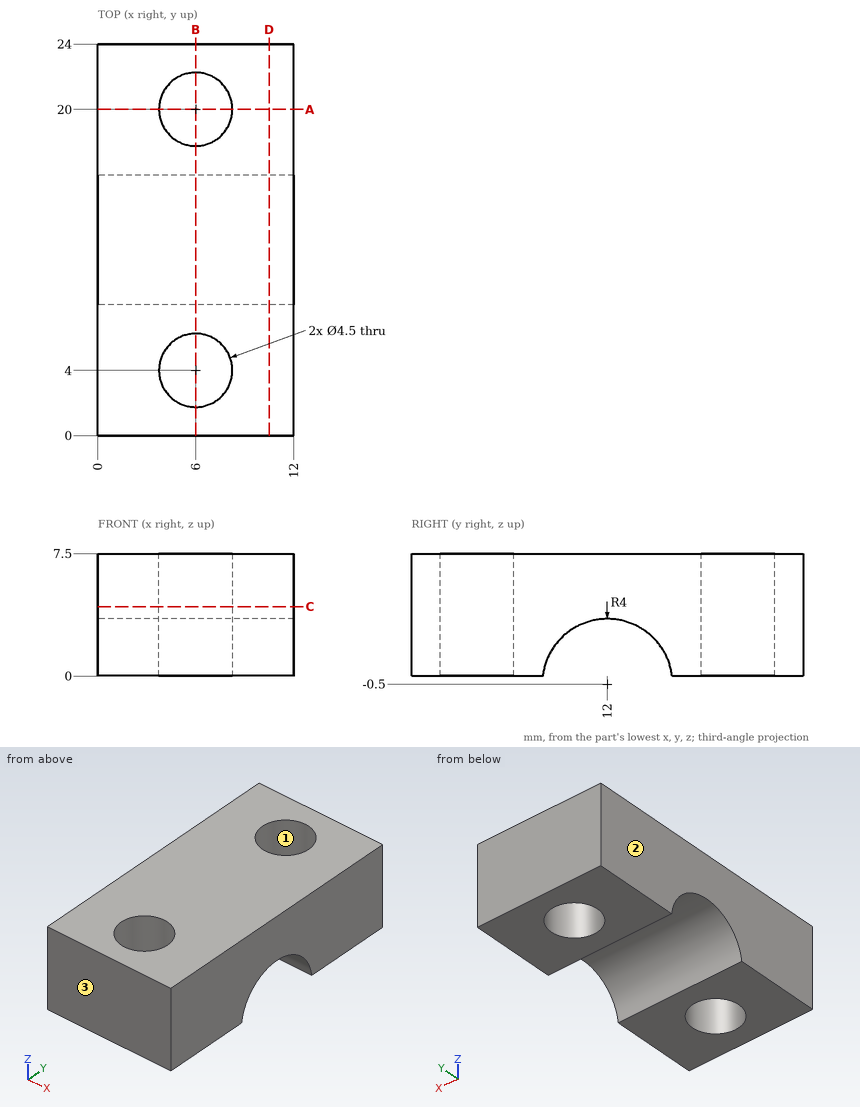
Check sheet for the drawn part. Datum: minimum x, y, z corner. Units: mm. Coordinates: 2 decimals unless noted, no trailing zeros. Order: outer loops, then holes, each group sorted by start corner. A loop starts at its lowest first (then second) coordinate and runs counter-clockwise, first axis right, second up. Notation, with made-up numbers: M -27,49 L -16,49 A12 ccw -16,66 Z; hole C 69,-34.75 d9. An arc over 180 degrees is marked long. One line per question, with ' | ' between items. Start each with the question number.
Item 1: Cross-section at C-C on z = 4.25. Enter the section's corners in (x, y), then the cut area to 3 significant figures.
Item 2: Cross-section at A-A on y = 20. Enter the section's corners in (x, z).
Item 3: Material ranges on L1, parallel to Y at x = 6, z = 5.25; L2, parallel to Y at x = 7.5, z = 5.25; L3, parallel to Y at x = 6, z = 2.25, recorded low to high. Write a range as [from, to].
Item 4: Cross-section at D-D on x = 10.5. Enter the section's corners in (y, z).
Item 5: Draft check along X on the marked faces 1, 2 and 3. Enter one of: pulls with the +X half, pulls with the -X half, needs draft (parallel to the pull), parting line crosses it, or undercut.
Item 6: Cross-section at B-B on x = 6. Enter the section's corners in (y, z).
Findings:
1) outline: M 0,0 L 12,0 L 12,24 L 0,24 Z; hole C 6,4 d4.5; hole C 6,20 d4.5 | area: 256 mm²
2) outline: M 0,0 L 3.75,0 L 3.75,7.5 L 0,7.5 Z; M 8.25,0 L 12,0 L 12,7.5 L 8.25,7.5 Z
3) L1: y = [0, 1.75], [6.25, 17.75], [22.25, 24] | L2: y = [0, 2.32], [5.68, 18.32], [21.68, 24] | L3: y = [0, 1.75], [6.25, 9.1], [14.9, 17.75], [22.25, 24]
4) outline: M 0,0 L 8.03,0 A4 cw 15.97,0 L 24,0 L 24,7.5 L 0,7.5 Z
5) face 1: undercut | face 2: pulls with the -X half | face 3: needs draft
6) outline: M 0,0 L 1.75,0 L 1.75,7.5 L 0,7.5 Z; M 6.25,0 L 8.03,0 A4 cw 15.97,0 L 17.75,0 L 17.75,7.5 L 6.25,7.5 Z; M 22.25,0 L 24,0 L 24,7.5 L 22.25,7.5 Z
